Design review of the part built by this model. Coordinates are the model's own, in mm. A direction names the side the tool comes from. Coordinates: 2 decimals unless noted, no trailing zeros. Loops run counter-clockwise (first coordinate to the right, second up) from the corner with the lowest first, then second, coordinate; pieces in that order, holes last. Notation, with made-up numbers: (77.25, 56.5) - (128.25, 56.5) arc R38 cw to (128.25, 95.5) - close; hole circle Ø8 at (-33, 43). An arc over 180 degrees is marked (long way). One line per question, with ' | ' between items.
from build123d import *

# Parameters (mm, degrees)
F1_DEPTH = 2
F3_DEPTH = 25


with BuildPart() as f1:
    # F0 (on Top) → F1 (new body)
    with BuildSketch(Plane.XY):
        with BuildLine():
            Line((4.281331, 10.132631), (3.535193, 8.366744))
            ThreePointArc((3.535193, 8.366744), (2.744845, 7.502753), (1.586626, 7.330533))
            ThreePointArc((1.586626, 7.330533), (0, 7.484539), (-1.586626, 7.330533))
            ThreePointArc((-1.586626, 7.330533), (-2.744845, 7.502753), (-3.535193, 8.366744))
            Line((-3.535193, 8.366744), (-4.281331, 10.132631))
            ThreePointArc((-4.281331, 10.132631), (-9.528654, 5.495885), (-10.914603, -1.368004))
            Line((-10.914603, -1.368004), (-9.178189, -1.150367))
            ThreePointArc((-9.178189, -1.150367), (-7.929849, -1.338514), (-7.132924, -2.317627))
            ThreePointArc((-7.132924, -2.317627), (-6.495191, -3.75), (-5.573586, -5.01848))
            ThreePointArc((-5.573586, -5.01848), (-5.124111, -6.198194), (-5.585341, -7.373362))
            Line((-5.585341, -7.373362), (-6.773725, -8.666986))
            ThreePointArc((-6.773725, -8.666986), (0, -11), (6.773725, -8.666986))
            Line((6.773725, -8.666986), (5.585341, -7.373362))
            ThreePointArc((5.585341, -7.373362), (5.124111, -6.198194), (5.573586, -5.01848))
            ThreePointArc((5.573586, -5.01848), (6.495191, -3.75), (7.132924, -2.317627))
            ThreePointArc((7.132924, -2.317627), (7.858216, -1.381697), (9.01341, -1.121806))
            Line((9.01341, -1.121806), (10.915781, -1.358574))
            ThreePointArc((10.915781, -1.358574), (10.978925, -0.680591), (11, 0))
            ThreePointArc((11, 0), (9.167733, 6.078872), (4.281331, 10.132631))
        make_face()
    extrude(amount=F1_DEPTH)

    # F2 (on face) → F3 (cut)
    with BuildSketch(Plane.XY.offset(2)):
        with BuildLine():
            ThreePointArc((1.572898, 7.333212), (0, 7.5), (-1.572898, 7.333212))
            ThreePointArc((-1.572898, 7.333212), (0, 7.484539), (1.572898, 7.333212))
        make_face()
        with BuildLine():
            Line((-1, 1), (-1, 6.161259))
            ThreePointArc((-1, 6.161259), (-4.413678, 4.413678), (-6.161259, 1))
            Line((-6.161259, 1), (-1, 1))
        make_face()
        with BuildLine():
            ThreePointArc((6.179031, 1), (4.426083, 4.426083), (1, 6.179031))
            Line((1, 6.179031), (1, 1))
            Line((1, 1), (6.179031, 1))
        make_face()
        with BuildLine():
            ThreePointArc((1.008042, -6.158178), (4.415323, -4.409561), (6.159489, -1))
            Line((6.159489, -1), (1, -1))
            Line((1, -1), (1.008042, -6.158178))
        make_face()
        with BuildLine():
            Line((-1, -1), (-6.177082, -1))
            ThreePointArc((-6.177082, -1), (-4.424723, -4.424723), (-1, -6.177082))
            Line((-1, -6.177082), (-1, -1))
        make_face()
    extrude(amount=-F3_DEPTH, mode=Mode.SUBTRACT)


solid = f1.part
Q1. Draft analysis for pull direction X (two halves, no side actions). For faces 5 (the cylindrical face through (0, -11, 1)), 6 (the cylindrical face through (0.022, 7.485, 0.986)), 7 (the flat face through (6.19, -8.03, 0.99)), state which applies: +X half, -X half, draft (parallel to the pull), parting line (faces both ways), or undercut.
Returned:
face 5: parting line | face 6: undercut | face 7: +X half
Q2. For pin 1 (0.6 mm diameter, centred on x = -3.5, z = 1, fed in from -Y); pin 2 (1 mm diameter, centred on x = 3.5, z = 0.5, fed in from +Y), all flat-tipped, find the tip position at first contact; note any pin that passes through.
Returned:
pin 1: stops at y = -10.52 | pin 2: stops at y = 9.47
Q3. Tool access review of faces 1 (the flat face through (-3.903, 9.237, 0.986)), 2 (the flat face through (-10.06, -1.26, 0.99)), 3 (the cylindrical face through (-6.506, -3.731, 0.986)), 4 (the flat face through (4, -1, 1)): name each direction out of +Z, -Z, +X, -X, +Y, -Y from which nothing blocks a thin tool from reaching the whole face with its end or side.
Returned:
face 1: +Z, -Z, +Y | face 2: +Z, -Z, -Y | face 3: +Z, -Z, -X | face 4: +Z, -Z
Q4. Take a section at D-D (y = 6.75). Give the boundary of the cut face in (x, z), plus the area to 3 significant figures.
Returned:
outline: (-8.69, 0) - (8.69, 0) - (8.69, 2) - (-8.69, 2) - close | area: 34.7 mm²
Q5. Take a section at A-A (y = -3.5). Give the boundary of the cut face in (x, z).
Returned:
outline: (-6.63, 0) - (-5.19, 0) - (-5.19, 2) - (-6.63, 2) - close; (-1, 0) - (1, 0) - (1, 2) - (-1, 2) - close; (5.17, 0) - (6.63, 0) - (6.63, 2) - (5.17, 2) - close
Q6. To check wall thickness, follow line 1 along Y through (x, z) = (2, 1.65); line 2 along Y through (x, z) = (-4, 1.2); line 3 along X through (y, z) = (1.5, 0.1). State the ranges of each line that lie inside material, in increasing order.
Returned:
line 1: y = -10.82 to -5.91, -1 to 1, 5.93 to 7.3 | line 2: y = -10.25 to -4.81, -1 to 1, 4.79 to 9.47 | line 3: x = -10.9 to -6.06, -1 to 1, 6.08 to 10.9
Q7. Take a section at B-B (x = -2). Give the boundary of the cut face in (y, z).
Returned:
outline: (-10.82, 0) - (-5.93, 0) - (-5.93, 2) - (-10.82, 2) - close; (-1, 0) - (1, 0) - (1, 2) - (-1, 2) - close; (5.91, 0) - (7.3, 0) - (7.3, 2) - (5.91, 2) - close
Q8. Take a section at C-C (z = 1.65). State how many separate pieces and enclosed holes the cut face has, plus the area to 3 significant figures.
Returned:
separate pieces: 1 | enclosed holes: 4 | area: 229 mm²
